Verification items for the finished model (mm, model axes). A direction names the side the tool comes from. Round coordinates to 2 decimals unless told otherwise and drop trailing zeros. Order: outer loops, then holes, each group sorted by start corner. A loop starts at its lowest first (then second) coordinate and runs counter-clockwise, first axis right, second up. Notation, with made-up numbers: M 39.5,46 L 93.5,46 A16 ccw 93.5,59 Z; hole C 15,50.25 d5. An arc over 180 degrees is marked long. Return JSON: item names as keys, results as strings. Group by question number.
from build123d import *

# Parameters (mm, degrees)
SKETCH1_W           = 25.4
SKETCH1_H           = 50.8
SKETCH1_W_2         = 20.32
SKETCH1_H_2         = 45.72
EXTRUDE_THIN1_DEPTH = 342.9
SKETCH2_R           = 2.0701
CUT_EXTRUDE1_DEPTH  = 51.8
LPATTERN1_COUNT     = 28
LPATTERN1_PITCH     = 25.4


with BuildPart() as part:
    # Sketch1 → Extrude-Thin1 (new body, symmetric)
    with BuildSketch(Plane.XY):
        Rectangle(SKETCH1_W, SKETCH1_H)
        Rectangle(SKETCH1_W_2, SKETCH1_H_2, mode=Mode.SUBTRACT)
    extrude(amount=EXTRUDE_THIN1_DEPTH, both=True)

    # Sketch2 → Cut-Extrude1 (cut, through all)
    with BuildSketch(Plane(origin=(0, 25.4, 0), x_dir=(1, 0, 0), z_dir=(0, 1, 0))):
        with Locations((0, -330.2)):
            Circle(SKETCH2_R)
    cut_extrude1 = extrude(amount=-CUT_EXTRUDE1_DEPTH, mode=Mode.SUBTRACT)

    # LPattern1: Cut-Extrude1 ×28
    with Locations(*[(0, 0, -i * LPATTERN1_PITCH) for i in range(1, LPATTERN1_COUNT)]):
        add(cut_extrude1, mode=Mode.SUBTRACT)


solid = part.part
1. Go/stop test with a flat-tipped pin: pin 1 (3.5 mm diameter, centred on x = 0, z = -101.6, fed in from +Y). Record where the tip stops, or that it passes through.
2. Cross-section at C-C (x = 6.25). Enter the section's corners in (y, z).
3. Cross-section at A-A (y = 13). Enter the section's corners in (x, z), plus the area to 3 significant figures.
4. Draft check along Y on faces 1 (the face through (-10.16, 0, 5)), 2 (the face through (0, -22.86, 5)), 3 (the face through (-10.4, 2, -342.9)), 4 (the face through (0, 25.4, 5)). Enter one of: +Y half, -Y half, draft (parallel to the pull), parting line (faces both ways), or undercut.
5. Access from +Z, -Z, +X, -X, +Y, -Y to the whole of each face (thin tool, end or side, straight path). Record for faces 5 (the face through (12.7, 0, 5)), 6 (the face through (10.16, 0, 5)).
6. Cross-section at B-B (z = 188). Enter the section's corners in (x, y).
7. Thickness scan on line 1 along Y through (x, z) = (1, 45); line 2 along X through (y, z) = (5, -26.5); line 3 along X through (y, z) = (24, 279). Record the ranges inside material, lowest first. Write a range as from..to.
Computed:
{
 "1": {"pin 1": "passes through"},
 "2": {"outline": "M -25.4,-342.9 L -22.86,-342.9 L -22.86,342.9 L -25.4,342.9 Z; M 22.86,-342.9 L 25.4,-342.9 L 25.4,342.9 L 22.86,342.9 Z"},
 "3": {"outline": "M -12.7,-342.9 L -10.16,-342.9 L -10.16,342.9 L -12.7,342.9 Z; M 10.16,-342.9 L 12.7,-342.9 L 12.7,342.9 L 10.16,342.9 Z", "area": "3,480 mm²"},
 "4": {"face 1": "undercut", "face 2": "undercut", "face 3": "draft", "face 4": "+Y half"},
 "5": {"face 5": "+Z, -Z, +X, +Y, -Y", "face 6": "+Z, -Z"},
 "6": {"outline": "M -12.7,-25.4 L 12.7,-25.4 L 12.7,25.4 L -12.7,25.4 Z; hole M -10.16,-22.86 L 10.16,-22.86 L 10.16,22.86 L -10.16,22.86 Z"},
 "7": {"line 1": "y = -25.4..-22.86, 22.86..25.4", "line 2": "x = -12.7..-10.16, 10.16..12.7", "line 3": "x = -12.7..-2.03, 2.03..12.7"}
}
